Can you work these out from the drawing? Everything is in mm from the part's minimum corner. A direction names the side the tool comes from. Coordinates: 2 decimals unless noted, no trailing zeros. Order: outer loops, then holes, each group sorted by start corner. A loop starts at its lowest first (then second) coordinate and runs counter-clockwise, first axis right, second up. Notation, with made-up numbers: (84.25, -34) -> (113.25, -34) arc R20 cw to (113.25, 2) -> close; hole circle Ø2 at (40.5, 12.5). An arc over 180 degrees is marked (long way). Use a Markdown table: item, result. Add a question column.
1) Will these pins go through, and if not, where does the flat tip stop? pin 1 Ø1.5 at (x, y) = (2, 17) entering from +Z (1 decimal); pin 2 Ø2 at (y, z) = (12, 3) entering from -X; pin 3 Ø3 at (x, y) = (1, 6) entering from -Z (1 decimal).
2) Which directions (+Z, -Z, +X, -X, +Y, -Y) give clear straight access to the entire face, cutting with the end or side of a thin tool? Please do the marked faces 4 and 5.
3) Thinking about a two-plate mould opening in Z: for the marked faces 1, 2 and 3, which applies, +Z half, -Z half, draft (parallel to the pull), parting line (faces both ways), or undercut?
4) If we section it at A-A (y = 8): Write out the boundary of the cut face in (x, z), plus the area to 3 significant figures.
5) If I drill on L1, parallel to Y at x = 2.75, z = 0.5; L2, parallel to Y at x = 4.5, z = 3.5; L3, parallel to Z at x = 2.5, y = 21.75, over which ranges is the centre line in solid material (lowest first)? Write a range as [from, to].
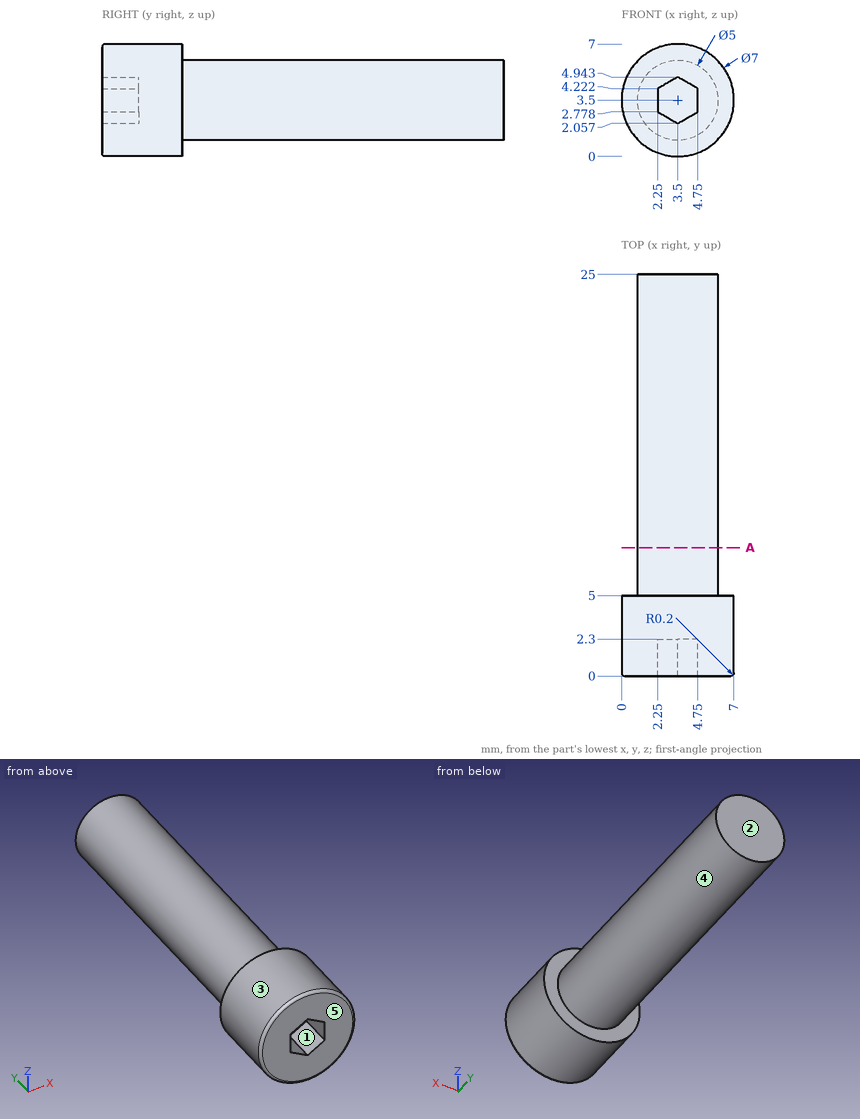
Answer sheet:
| question | item | result |
|---|---|---|
| 1 | pin 1 | z = 5.9 |
| 1 | pin 2 | x = 1 |
| 1 | pin 3 | z = 0.3 |
| 2 | face 4 | +Y |
| 2 | face 5 | +Z, -Z, +X, -X, -Y |
| 3 | face 1 | undercut |
| 3 | face 2 | draft |
| 3 | face 3 | parting line |
| 4 | outline | circle Ø5 at (3.5, 3.5) |
| 4 | area | 19.6 mm2 |
| 5 | L1 | [0, 5] |
| 5 | L2 | [2.3, 25] |
| 5 | L3 | [1.21, 5.79] |
